```python
from build123d import *

# Parameters (mm, degrees)
CYLINDER012029001058_R       = 1.75
CYLINDER012029001058_DEPTH   = 6
CYLINDER012029001059_R       = 6.88
CYLINDER012029001059_DEPTH   = 2
CYLINDER012029001060_R       = 1.75
CYLINDER012029001060_DEPTH   = 6
BOX015001051_W               = 20
BOX015001051_H               = 20
BOX015001051_DEPTH           = 28
BOX015001051_PLACEMENT_ANGLE = 45
BOX015001050_W               = 37.15
BOX015001050_H               = 242.75
BOX015001050_DEPTH           = 14.95
BOX015001048_W               = 50
BOX015001048_H               = 246
BOX015001048_DEPTH           = 14.95
BOX015001049_W               = 50
BOX015001049_H               = 246
BOX015001049_DEPTH           = 3.75
CYLINDER012029001061_R       = 6.88
CYLINDER012029001061_DEPTH   = 2


with BuildPart() as cylinder012029001058:
    # Cylinder012029001058 → Cylinder012029001058 (new body)
    with BuildSketch(Plane(origin=(21.63, 233.64, -2), x_dir=(1, 0, 0), z_dir=(0, 0, 1))):
        Circle(CYLINDER012029001058_R)
    extrude(amount=CYLINDER012029001058_DEPTH)


with BuildPart() as cylinder012029001059:
    # Cylinder012029001059 → Cylinder012029001059 (new body)
    with BuildSketch(Plane(origin=(21.63, 233.64, -2), x_dir=(1, 0, 0), z_dir=(0, 0, 1))):
        Circle(CYLINDER012029001059_R)
    extrude(amount=CYLINDER012029001059_DEPTH)


with BuildPart() as cylinder012029001060:
    # Cylinder012029001060 → Cylinder012029001060 (new body)
    with BuildSketch(Plane(origin=(21.63, 26.63, -2), x_dir=(1, 0, 0), z_dir=(0, 0, 1))):
        Circle(CYLINDER012029001060_R)
    extrude(amount=CYLINDER012029001060_DEPTH)


with BuildPart() as cube045:
    # Box015001051 → Box015001051 (new body)
    with BuildSketch(Plane.XY):
        with Locations((10, 10)):
            Rectangle(BOX015001051_W, BOX015001051_H)
    extrude(amount=BOX015001051_DEPTH)


with BuildPart() as cube045_1:
    # Box015001051 placement: moved
    add(cube045.part.moved(Location((0, -14.1422, 17.8921))).rotate(Axis((0, -14.1422, 17.8921), (-1, 0, 0)), BOX015001051_PLACEMENT_ANGLE))


with BuildPart() as cube003:
    # Box015001050 → Box015001050 (new body)
    with BuildSketch(Plane(origin=(12.85, 0, 3.75), x_dir=(1, 0, 0), z_dir=(0, 0, 1))):
        with Locations((18.575, 121.375)):
            Rectangle(BOX015001050_W, BOX015001050_H)
    extrude(amount=BOX015001050_DEPTH)


with BuildPart() as cut003053:
    # Box015001048 → Box015001048 (new body)
    with BuildSketch(Plane.XY.offset(3.75)):
        with Locations((25, 123)):
            Rectangle(BOX015001048_W, BOX015001048_H)
    extrude(amount=BOX015001048_DEPTH)

    # Cut003052: cut Cube003
    add(cube003.part, mode=Mode.SUBTRACT)

    # Cut003053: cut Cube045
    add(cube045_1.part, mode=Mode.SUBTRACT)


with BuildPart() as fusion001019007005:
    # Box015001049 → Box015001049 (new body)
    with BuildSketch(Plane.XY):
        with Locations((25, 123)):
            Rectangle(BOX015001049_W, BOX015001049_H)
    extrude(amount=BOX015001049_DEPTH)

    # Fusion001019007005: union Cut003053
    add(cut003053.part)


with BuildPart() as cut003:
    # Cylinder012029001061 → Cylinder012029001061 (new body)
    with BuildSketch(Plane(origin=(21.63, 26.63, -2), x_dir=(1, 0, 0), z_dir=(0, 0, 1))):
        Circle(CYLINDER012029001061_R)
    extrude(amount=CYLINDER012029001061_DEPTH)

    # Fusion001019007004: union Fusion001019007005
    add(fusion001019007005.part)

    # Cut003054: cut Cylinder012029001060
    add(cylinder012029001060.part, mode=Mode.SUBTRACT)

    # Fusion001019007003: union Cylinder012029001059
    add(cylinder012029001059.part)

    # Cut003: cut Cylinder012029001058
    add(cylinder012029001058.part, mode=Mode.SUBTRACT)


with BuildPart() as part_mirroring:
    # Part__Mirroring: instance of Cut003
    add(cut003.part.mirror(Plane(origin=(126, 0, 0), x_dir=(0, -1, 0), z_dir=(1, 0, 0))))


solid = part_mirroring.part
```
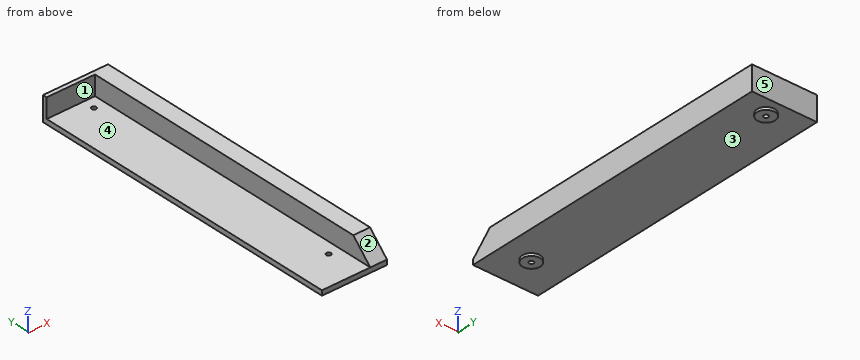
Check sheet for the modelled part. Datum: model origin and axes. Units: mm. Face numbers are marked on the shaded views. A direction names the side the tool comes from. Round coordinates to 2 decimals unless told otherwise and drop trailing zeros. Order: outer loops, then holes, each group sorted by start corner. A loop starts at its lowest first (then second) coordinate and runs counter-clockwise, first axis right, second up. Notation, with made-up numbers: M 31,61 L 84,61 A16 cw 84,69 Z; hole C 20.5,-5 d7. An arc over 180 degrees is marked long. Answer in a Markdown table with one row per item.
(1) Section check D-D on x = 226.5. Record the boundary of the cut face in (y, z).
Findings:
| item | result |
|---|---|
| outline | M 0,0 L 20.94,0 L 20.94,-2 L 32.32,-2 L 32.32,0 L 227.95,0 L 227.95,-2 L 239.33,-2 L 239.33,0 L 246,0 L 246,18.7 L 242.75,18.7 L 242.75,3.75 L 0,3.75 Z |
(2) Material ranges on line 1 along Y through (x, z) = (230.37, 0.75); line 2 along X through (y, z) = (233.64, 1.05); line 3 along Z through (x, y) = (236.5, 187), recorded low to high. Write a range as from..to.
Findings:
| item | result |
|---|---|
| line 1 | y = 0..24.88, 28.38..231.89, 235.39..246 |
| line 2 | x = 202..228.62, 232.12..252 |
| line 3 | z = 0..3.75 |
(3) Set-up check for the marked faces 1 and 2: record each of +Z, -Z, +X, -X, +Y, -Y from which the full face is reachable in a straight line by a thin tool's end or side.
Findings:
| item | result |
|---|---|
| face 1 | +Z, -X, -Y |
| face 2 | +Z, +X, -X, -Y |
(4) Section check A-A on x = 209. Record the boundary of the cut face in (y, z).
Findings:
| item | result |
|---|---|
| outline | M 0,0 L 246,0 L 246,18.7 L 242.75,18.7 L 242.75,3.75 L 0,3.75 Z |
(5) Section check C-C on x = 245.5. Record the boundary of the cut face in (y, z), plus the area to 3 significant figures.
Findings:
| item | result |
|---|---|
| outline | M 0,0 L 246,0 L 246,18.7 L 14.95,18.7 L 0,3.75 Z |
| area | 4,490 mm^2 |
(6) Gauge pin test, flat ends, axial feed: pin 1 (25 mm diameter, centred on x = 223, y = 156, fed in from -Z); pin 2 (4.5 mm diameter, centred on x = 230.37, y = 26.63, fed in from +Z); pin 3 (6 mm diameter, centred on x = 238, z = 11.5, fed in from -Y). Record the tip position at first contact, or that the pin passes through.
Findings:
| item | result |
|---|---|
| pin 1 | stops at z = 0 |
| pin 2 | stops at z = 3.75 |
| pin 3 | stops at y = 4.98 |
(7) Section check B-B on y = 78. Record the boundary of the cut face in (x, z), plus the area to 3 significant figures.
Findings:
| item | result |
|---|---|
| outline | M 202,0 L 252,0 L 252,18.7 L 239.15,18.7 L 239.15,3.75 L 202,3.75 Z |
| area | 380 mm^2 |
(8) Draft check along Y on the marked faces 3, 4 and 5. Enter one of: +Y half, -Y half, draft (parallel to the pull), parting line (faces both ways), or undercut.
Findings:
| item | result |
|---|---|
| face 3 | undercut |
| face 4 | draft |
| face 5 | +Y half |
